from build123d import *

# Parameters (mm, degrees)
SKETCH_R        = 1.65
PAD_DEPTH       = 6.5
POCKET_DEPTH    = 2.5
PAD001_DEPTH    = 47.2
CHAMFER_SIZE    = 1
PAD002_DEPTH    = 52.25
SKETCH004_R     = 2.475
POCKET001_DEPTH = 15
PAD003_DEPTH    = 5
SKETCH006_R     = 3.45
SKETCH006_R_2   = 2.45
PAD004_DEPTH    = 3
CHAMFER001_SIZE = 3


with BuildPart() as part:
    # Sketch → Pad (new body)
    with BuildSketch(Plane.XY):
        with BuildLine():
            ThreePointArc((-3, 0), (0, -3), (3, 0))
            Line((3, 0), (3, 26.125))
            Line((3, 26.125), (26.125, 26.125))
            Line((26.125, -26.125), (26.125, 26.125))
            Line((-26.125, -26.125), (26.125, -26.125))
            Line((-26.125, 26.125), (-26.125, -26.125))
            Line((-26.125, 26.125), (-3, 26.125))
            Line((-3, 0), (-3, 26.125))
        make_face()
        with Locations((-15.5, -15.5)):
            Circle(SKETCH_R, mode=Mode.SUBTRACT)
        with Locations((15.5, -15.5)):
            Circle(SKETCH_R, mode=Mode.SUBTRACT)
        with Locations((15.5, 15.5)):
            Circle(SKETCH_R, mode=Mode.SUBTRACT)
        with Locations((-15.5, 15.5)):
            Circle(SKETCH_R, mode=Mode.SUBTRACT)
    extrude(amount=PAD_DEPTH)

    # Sketch001 (on Face14 of Pad) → Pocket (cut)
    with BuildSketch(Plane.XY.offset(6.5)):
        with BuildLine():
            ThreePointArc((-11.1, 0), (0, -11.1), (11.1, 0))
            Line((11.1, 0), (11.1, 26.125))
            Line((-11.1, 26.125), (11.1, 26.125))
            Line((-11.1, 0), (-11.1, 26.125))
        make_face()
    extrude(amount=-POCKET_DEPTH, mode=Mode.SUBTRACT)

    # Sketch002 (on Face6 of Pocket) → Pad001 (join)
    with BuildSketch(Plane.XY.offset(6.5)):
        Polygon((-26.125, -26.125), (-26.125, 26.125), (-21.125, 26.125), (-21.125, -21.125), (21.125, -21.125), (21.125, 26.125), (26.125, 26.125), (26.125, -26.125), align=None)
    extrude(amount=PAD001_DEPTH)

    # Chamfer
    chamfer_edges = [part.edges().sort_by_distance(p)[0] for p in [
        (3, 26.125, 2),
        (11.1, 26.125, 5.25),
        (-3, 26.125, 2),
        (-11.1, 26.125, 5.25),
    ]]
    chamfer(chamfer_edges, length=CHAMFER_SIZE)

    # Sketch003 (on Face10 of Chamfer) → Pad002 (join)
    with BuildSketch(Plane(origin=(0, 26.125, 0), x_dir=(-1, 0, 0), z_dir=(0, 1, 0))):
        Polygon((-26.125, 53.7), (-23.5, 59.7), (-23.5, 74.7), (-16.5, 74.7), (-16.5, 59.7), (-21.125, 53.7), align=None)
        Polygon((26.125, 53.7), (23.5, 59.7), (23.5, 74.7), (16.5, 74.7), (16.5, 59.7), (21.125, 53.7), align=None)
    extrude(amount=-PAD002_DEPTH)

    # Sketch004 (on Face32 of Pad002) → Pocket001 (cut)
    with BuildSketch(Plane.XY.offset(74.7)):
        with Locations((-20, 10)):
            Circle(SKETCH004_R)
        with Locations((-20, -10)):
            Circle(SKETCH004_R)
        with Locations((20, -10)):
            Circle(SKETCH004_R)
        with Locations((20, 10)):
            Circle(SKETCH004_R)
    extrude(amount=-POCKET001_DEPTH, mode=Mode.SUBTRACT)

    # Sketch005 (on Face6 of Pocket001) → Pad003 (join)
    with BuildSketch(Plane.XZ.offset(26.125)):
        Polygon((-16.5, 59.7), (16.5, 59.7), (21.125, 53.7), (-21.125, 53.7), align=None)
    extrude(amount=-PAD003_DEPTH)

    # Sketch006 (on Face17 of Pad003) → Pad004 (join)
    with BuildSketch(Plane.XY.offset(74.7)):
        with Locations((-20, 0)):
            Circle(SKETCH006_R)
        with Locations((20, 0)):
            Circle(SKETCH006_R_2)
    extrude(amount=PAD004_DEPTH)

    # Chamfer001
    chamfer001_edges = [part.edges().sort_by_distance(p)[0] for p in [
        (26.125, 0, 0),
        (15.0625, 26.125, 0),
        (-15.0625, 26.125, 0),
        (-26.125, 0, 0),
        (0, -26.125, 0),
    ]]
    chamfer(chamfer001_edges, length=CHAMFER001_SIZE)


solid = part.part
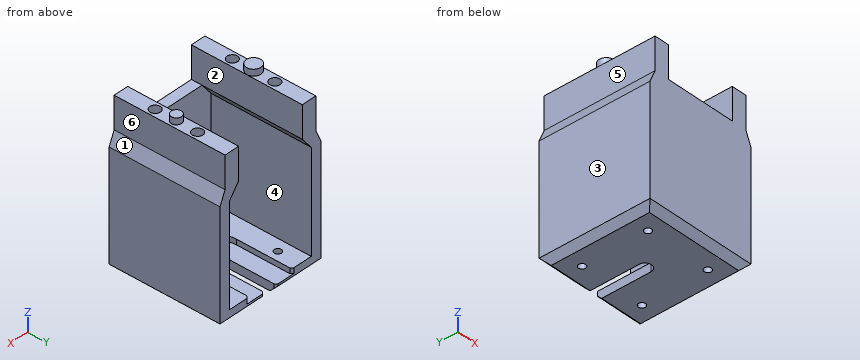
Could you check a few things on this model? Use its own coordinates, in mm. Face numbers are marked on the shaded views. A direction names the side the tool comes from. Give positions to 0.01 mm unless a question says otherwise; leave off trailing zeros. Order: outer loops, then holes, each group sorted by start corner. A loop starts at its lowest first (then second) coordinate and runs counter-clockwise, first axis right, second up. Notation, with made-up numbers: (59, 36) - (82, 36) arc R32 ccw to (82, 73) - close; hole circle Ø2 at (87.25, 43.25). An arc over 180 degrees is marked (long way). Return JSON: item names as keys, results as strings. Group by question number.
Q1. Suppose I cut it at B-B, the plane y = -15.5. Please give me the cut outline in (x, z) (3 decimals).
Q2. Thinking about a two-plate mould opening in X: for the marked faces 1, 2 and 3, which applies, pulls with the +X half, pulls with the -X half, needs draft (parallel to the pull), parting line crosses it, or undercut?
Q3. Which directions (+Z, -Z, +X, -X, +Y, -Y) give clear straight access to the entire face, cutting with the end or side of a thin tool? Please do the marked faces 4, 5 and 6.
Q4. Please list where these lines run through material, in increasing order: line 1 along Y through (x, z) = (-15.5, 4.5) (3 decimals); line 2 along X through (y, z) = (1, 74.5); line 3 along Y through (x, z) = (-17, 5.5) (3 decimals). Write a range as [from, to].
Q5. Suppose I cut it at D-D, the plane x = 0. Please give me the cut outline in (y, z) (3 decimals), and give its area (3 significant figures).
Q6. Suppose I cut it at C-C, the plane y = 15.5. State how many separate pieces and enclosed holes the cut face has, and give its area (3 significant figures).
Q7. Will these pins go through, and if not, where does the flat tip stop? pin 1 Ø12.5 at (x, y) = (-7.5, 11) entering from +Z; pin 2 Ø2 at (y, z) = (16, 1) entering from -X (3 decimals); pin 3 Ø6.5 at (x, y) = (20, 10) entering from +Z; pin 4 Ø4.5 at (y, z) = (13.5, 2) entering from +X (3 decimals).
Q8. Suppose I cut it at A-A, the plane z = 62.5. Please give me the cut outline in (x, y) (3 decimals), and give its area (3 significant figures).
Resolved:
{
 "1": {"outline": "(-26.125, 3) - (-23.125, 0) - (-17.15, 0) - (-17.15, 6.5) - (-21.125, 6.5) - (-21.125, 53.7) - (-16.5, 59.7) - (-16.5, 74.7) - (-23.5, 74.7) - (-23.5, 59.7) - (-26.125, 53.7) - close; (-13.85, 0) - (13.85, 0) - (13.85, 6.5) - (-13.85, 6.5) - close; (16.5, 59.7) - (21.125, 53.7) - (21.125, 6.5) - (17.15, 6.5) - (17.15, 0) - (23.125, 0) - (26.125, 3) - (26.125, 53.7) - (23.5, 59.7) - (23.5, 74.7) - (16.5, 74.7) - close"},
 "2": {"face 1": "pulls with the +X half", "face 2": "undercut", "face 3": "pulls with the -X half"},
 "3": {"face 4": "+Y", "face 5": "+Z, -X, +Y, -Y", "face 6": "+Z, +X, +Y, -Y"},
 "4": {"line 1": "y = [-26.125, -17.15], [-13.85, 13.85], [17.15, 26.125]", "line 2": "x = [-23.5, -16.5], [16.5, 23.5]", "line 3": "y = [-26.125, -16.187], [-14.813, 14.813], [16.187, 26.125]"},
 "5": {"outline": "(-26.125, 3) - (-23.125, 0) - (-3, 0) - (-3, 4) - (-11.1, 4) - (-11.1, 6.5) - (-21.125, 6.5) - (-21.125, 59.7) - (-26.125, 59.7) - close", "area": "392 mm2"},
 "6": {"separate pieces": "4", "enclosed holes": "0", "area": "962 mm2"},
 "7": {"pin 1": "stops at z = 6.5", "pin 2": "stops at x = -25.125", "pin 3": "stops at z = 74.7", "pin 4": "stops at x = 26.125"},
 "8": {"outline": "(-23.5, -26.125) - (-16.5, -26.125) - (-16.5, 26.125) - (-23.5, 26.125) - close; (16.5, -26.125) - (23.5, -26.125) - (23.5, 26.125) - (16.5, 26.125) - close; hole circle Ø4.95 at (-20, -10); hole circle Ø4.95 at (-20, 10); hole circle Ø4.95 at (20, -10); hole circle Ø4.95 at (20, 10)", "area": "655 mm2"}
}
